from build123d import *

# Parameters (mm, degrees)
F0_R     = 8
F1_DEPTH = 101.6
F2_R     = 8.789608
F3_DEPTH = 7.62


with BuildPart() as f1:
    # F0 (on Top) → F1 (new body)
    with BuildSketch(Plane.XY):
        Circle(F0_R)
    extrude(amount=F1_DEPTH)

    # F2 (on Front) → F3 (join, symmetric)
    with BuildSketch(Plane.XZ):
        with Locations((0, 108.582966)):
            Circle(F2_R)
    extrude(amount=F3_DEPTH, both=True)


solid = f1.part
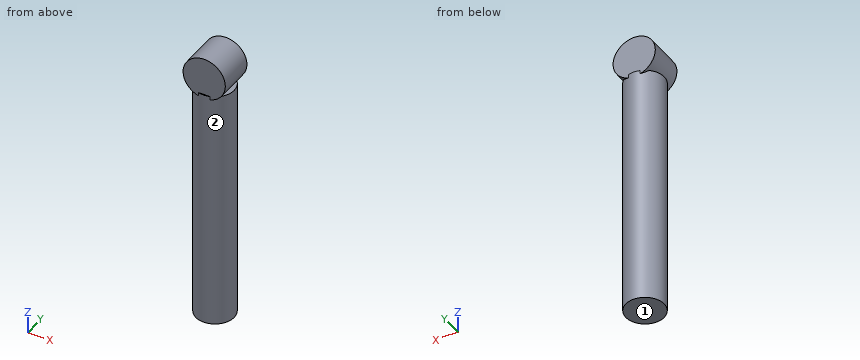
Work out the finished part from the listing and answer in its coordinate system (mm). Face numbers are marked on the shaded views. A direction names the side the tool comes from. Give positions to 0.01 mm unless a question says otherwise; leave off trailing zeros. Order: outer loops, then holes, each group sorted by start corner. A loop starts at its lowest first (then second) coordinate and runs counter-clockwise, first axis right, second up. Notation, with made-up numbers: (64, 85.25) -> (70, 85.25) arc R16 ccw to (70, 113.25) -> close; hole circle Ø5 at (65.25, 40.5). An arc over 180 degrees is marked (long way). One line per item, written item: value.
Item 1: Find section C-C, the plane z = 46.5. Give the vertices of the cut face in (x, y), plus the area to 3 significant figures.
Answer sheet:
outline: circle Ø16 at (0, 0)
area: 201 mm²
Item 2: A tool of negligible diameter and unlimited length cuts with its end or side. For the marked faces 1 and 2, from which of +Z, -Z, +X, -X, +Y, -Y can it reach the whole face along a straight path? Write none if from no direction.
Answer sheet:
face 1: -Z, +X, -X, +Y, -Y
face 2: -Z
Item 3: Flat-ended cylindrical pins translate along their axes: P1, Ø2, axis at x = -2.5, z = 18, coming from the +Y side; P2, Ø0.8, axis at x = -7, y = -1, coming from the +Z side; P3, Ø3, axis at x = 1.5, y = 2.5, coming from the -Z side; P4, Ø4, axis at y = 6.5, z = 52.5, coming from the -X side. Find the tip coordinate at first contact, or state that the pin passes through.
Answer sheet:
P1: y = 7.86
P2: z = 114.39
P3: z = 0
P4: x = -6.61
Item 4: Find section B-B, the plane y = 0. Give the vertices of the cut face in (x, z).
Answer sheet:
outline: (-8, 0) -> (8, 0) -> (8, 101.6) -> (5.34, 101.6) arc R8.79 ccw (long way) to (-5.34, 101.6) -> (-8, 101.6) -> close
Item 5: Straight lines are drawn through the part: probe 1 along Y at (x, z) = (4.5, 104.5); probe 2 along X at (y, z) = (0, 50); probe 3 along Y at (x, z) = (-0.5, 88). For each, find the intervals that lie inside material, in ascending order.
Answer sheet:
probe 1: -7.62 to 7.62
probe 2: -8 to 8
probe 3: -7.98 to 7.98
Item 6: Find section A-A, the plane x = 6.5. Give the vertices of the cut face in (y, z), plus the area to 3 significant figures.
Answer sheet:
outline: (-7.62, 102.67) -> (7.62, 102.67) -> (7.62, 114.5) -> (-7.62, 114.5) -> close; (-4.66, 0) -> (4.66, 0) -> (4.66, 101.6) -> (-4.66, 101.6) -> close
area: 1,130 mm²
